from build123d import *

# Parameters (mm, degrees)
F0_R     = 11.7502279649
F1_DEPTH = 25.4
F2_DEPTH = 25.4
F3_W     = 50.8
F3_H     = 24.9936
F4_DEPTH = 25.4
F5_R     = 5.08
F6_R     = 5.08


with BuildPart() as f1:
    # F0 (on Front) → F1 (new body)
    with BuildSketch(Plane.XZ):
        with BuildLine():
            ThreePointArc((-21.9455999374, 0), (-52.740892143, 28.8858766168), (-60.0455999374, -12.7))
            Line((-60.0455999374, -12.7), (41.5544000626, -12.7))
            Line((41.5544000626, -12.7), (41.5544000626, 0))
            Line((41.5544000626, 0), (-21.9455999374, 0))
        make_face()
        with Locations((-45.1517072222, 6.1183218543)):
            Circle(F0_R, mode=Mode.SUBTRACT)
    extrude(amount=F1_DEPTH)

    # F2 (add): a face of the model
    f2_faces = [f1.faces().sort_by_distance(p)[0] for p in [
        (-23.82283695, 0, 2.1208901059),
    ]]
    extrude(f2_faces, amount=F2_DEPTH)

    # F3 (on face) → F4 (cut)
    with BuildSketch(Plane.XY):
        with Locations((16.1544000626, -0.4653680826)):
            Rectangle(F3_W, F3_H)
    extrude(amount=-F4_DEPTH, mode=Mode.SUBTRACT)

    # F5
    f5_edges = [f1.edges().sort_by_distance(p)[0] for p in [
        (41.5544, 12.031432, -6.35),
        (41.5544, 25.4, -6.35),
    ]]
    fillet(f5_edges, radius=F5_R)

    # F6
    f6_edges = [f1.edges().sort_by_distance(p)[0] for p in [
        (41.5544, -12.962168, -6.35),
        (41.5544, -25.4, -6.35),
    ]]
    fillet(f6_edges, radius=F6_R)


solid = f1.part
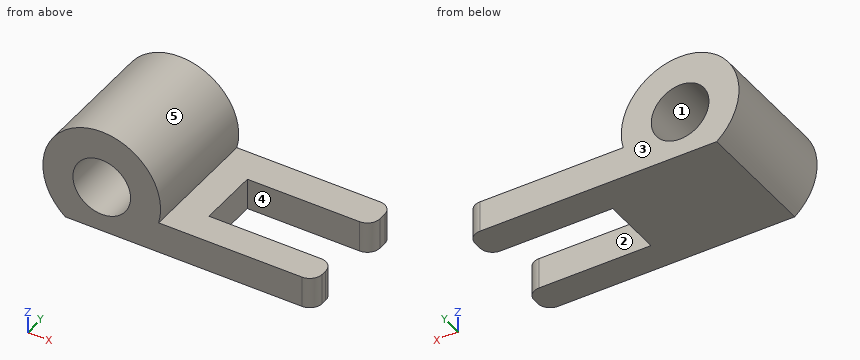
The listing builds one solid part. Answer for the finished solid, in the listing's coordinates (mm). Face numbers are marked on the shaded views. A direction names the side the tool comes from. Give positions to 0.01 mm unless a question says otherwise; leave off trailing zeros. Loops run counter-clockwise (first coordinate to the right, second up) from the corner with the lowest first, then second, coordinate; pieces in that order, holes last.
Item 1: Determine the mould class of the marked faces 1, 2 and 3 for opening direction Y: +Y half, -Y half, draft (parallel to the pull), parting line (faces both ways), or undercut.
Derived:
face 1: draft
face 2: undercut
face 3: +Y half
Item 2: Find the intervals of material crossed by line 1 along Y through (x, z) = (24, -3.5); line 2 along Z through (x, y) = (-11, 3); line 3 along X through (y, z) = (1, 5.5), in increasing order.
Derived:
line 1: y = -25.4 to -12.96, 12.03 to 25.4
line 2: z = -12.7 to 0
line 3: x = -69.14 to -56.89, -33.42 to -21.16
Item 3: Each of these flat-tipped pins is pushed along its axis until it touches: pin 1 Ø5 at (x, y) = (-27, 18.5) entering from +Z; pin 2 Ø5 at (y, z) = (-19.5, -5) entering from -X; pin 3 Ø5 at (y, z) = (-18.5, -1) entering from -X; pin 4 Ø21 at (x, z) = (-45.15, 6.12) entering from +Y. Where does it stop, or does it pass through?
Derived:
pin 1: stops at z = 24.31
pin 2: stops at x = -67.55
pin 3: stops at x = -68.7
pin 4: passes through
Item 4: A cutting plane is placed at A-A (x = 31). Give the vertices of the cut face in (y, z).
Derived:
outline: (-25.4, -12.7) - (-12.96, -12.7) - (-12.96, 0) - (-25.4, 0) - close; (12.03, -12.7) - (25.4, -12.7) - (25.4, 0) - (12.03, 0) - close
Item 5: A cutting plane is placed at B-B (z = 8). Give the vertices of the cut face in (x, y).
Derived:
outline: (-69.08, -25.4) - (-56.75, -25.4) - (-56.75, 25.4) - (-69.08, 25.4) - close; (-33.55, -25.4) - (-21.23, -25.4) - (-21.23, 25.4) - (-33.55, 25.4) - close
Item 6: A cutting plane is placed at C-C (y = -15). Give the vertices of the cut face in (x, z), then the cut area to 3 significant figures.
Derived:
outline: (-60.05, -12.7) - (40.54, -12.7) - (40.54, 0) - (-21.95, 0) arc R24 ccw (long way) to start; hole circle Ø23.5 at (-45.15, 6.12)
area: 2,100 mm2
Item 7: A cutting plane is placed at D-D (z = -3). Give the vertices of the cut face in (x, y), then the cut area to 3 significant figures.
Derived:
outline: (-67.35, -25.4) - (-52.56, -25.4) - (-52.56, 25.4) - (-67.35, 25.4) - close; (-37.74, -25.4) - (36.47, -25.4) arc R5.08 ccw to (41.55, -20.32) - (41.55, -18.04) arc R5.08 ccw to (36.47, -12.96) - (-9.25, -12.96) - (-9.25, 12.03) - (36.47, 12.03) arc R5.08 ccw to (41.55, 17.11) - (41.55, 20.32) arc R5.08 ccw to (36.47, 25.4) - (-37.74, 25.4) - close
area: 3,490 mm2
Item 8: A tool of negligible diameter and unlimited length cuts with its end or side. For the marked faces 4 and 5, from which of +Z, -Z, +X, -X, +Y, -Y can it reach the whole face along a straight path? Write none if from no direction.
Derived:
face 4: +Z, -Z, +X
face 5: +Y, -Y
